Could you check a few things on this drawing? It's one solid part, dimensions in mm from its lowest x, y, z. Coordinates: 2 decimals unless noted, no trailing zeros. Order: outer loops, then holes, each group sorted by start corner. A loop starts at its lowest first (then second) coordinate and runs counter-clockwise, first axis right, second up. Notation, with made-up numbers: M -5.75,-20 L 50.25,-20 A20 ccw 50.25,-10 Z; hole C -15.5,85.5 d2. An arc over 180 degrees is marked long. Answer as CSV lines item,"result". Start each with the question number.
1. I need wall thicknesses on line 1 along X through (y, z) = (12.5, 99); line 2 along X through (y, z) = (15, 107.5); line 3 along Z through (x, y) = (146, 4.5) (1 decimal). Which ranges of each line are inside material? Lowest first, please. Write a range as from..to.
2. If we section it at A-A (y = 13.25): List the corners of the cut face in (x, z) for me (1 decimal).
3. Will these pins go through, and if not, where does the flat tip stop? pin 1 (6 mm diameter, centred on y = 19, z = 84.5, fed in from -X); pin 2 (10 mm diameter, centred on x = 191, z = 26.5, fed in from -Y); pin 3 (4 mm diameter, centred on x = 175, y = 4.5, fed in from -Z); pin 4 (10 mm diameter, centred on y = 5, z = 180, fed in from -X).
4. If we mould it in two halves opening along Y, with no side actions, what happens to the marked faces 1 and 2? For each: released by +Y, released by -Y, zero draft, split by the parting line, or undercut.
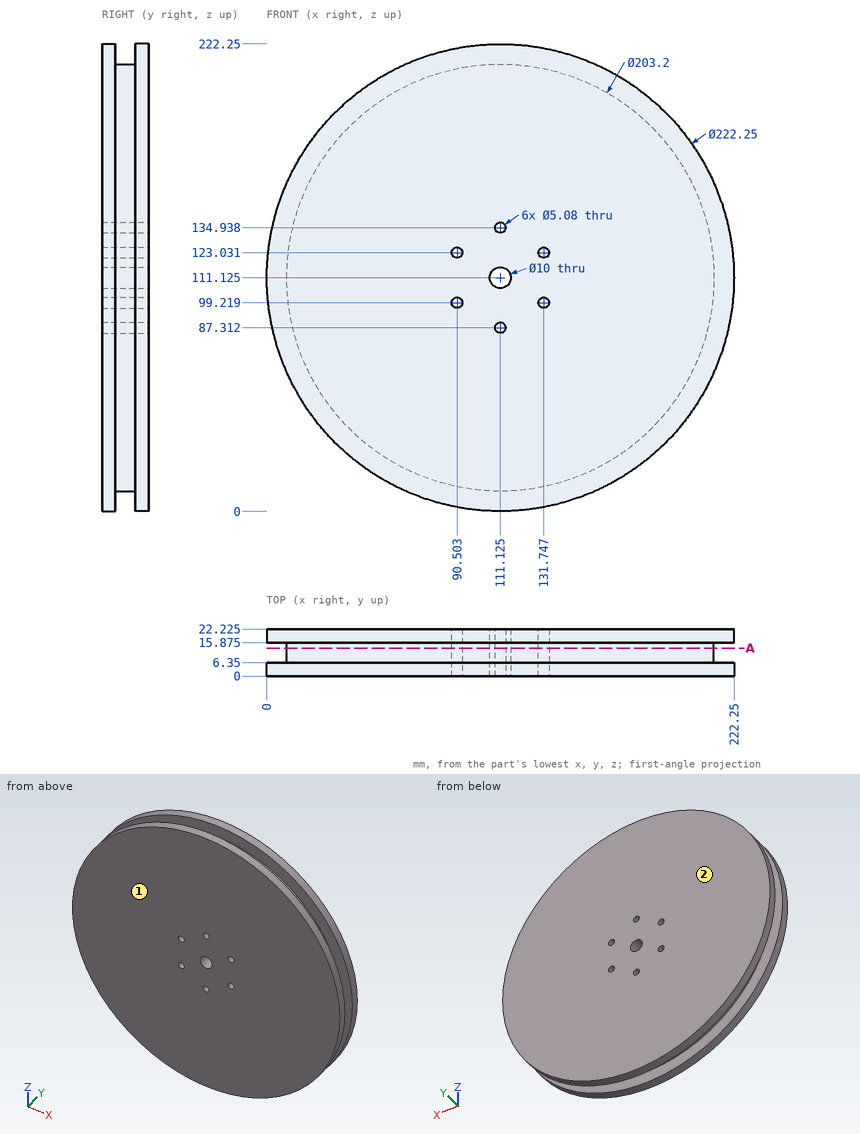
Solved:
1,line 1,"10.25..87.97, 93.03..129.22, 134.28..212"
1,line 2,"9.59..107.68, 114.57..212.66"
1,line 3,"5.6..216.6"
2,outline,"C 111.1,111.1 d203.2; hole C 90.5,99.2 d5.1; hole C 90.5,123 d5.1; hole C 111.1,111.1 d10; hole C 111.1,87.3 d5.1; hole C 111.1,134.9 d5.1; hole C 131.7,99.2 d5.1; hole C 131.7,123 d5.1"
3,pin 1,"x = 2.54"
3,pin 2,"through"
3,pin 3,"z = 18.82"
3,pin 4,"x = 20.19"
4,face 1,"released by -Y"
4,face 2,"released by +Y"
